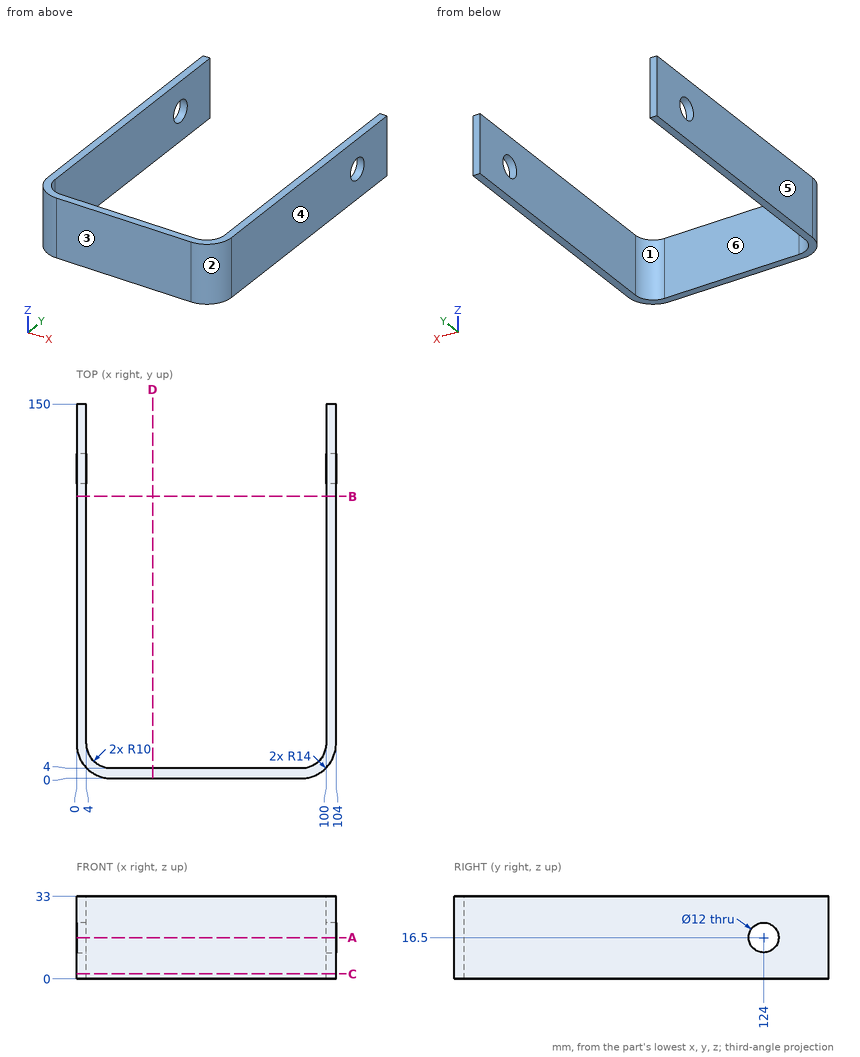
Here's the drawing with two shaded views (mm, measured from the low corner). I have some questions. A direction names the side the tool comes from. Give positions to 0.01 mm unless a question says otherwise; leave off trailing zeros. Order: outer loops, then holes, each group sorted by start corner. A loop starts at its lowest first (then second) coordinate and runs counter-clockwise, first axis right, second up. Notation, with made-up numbers: (60.25, 56) - (79.25, 56) arc R12 cw to (79.25, 75) - close; hole circle Ø8 at (20, 65). An arc over 180 degrees is marked (long way). Use a Markdown table: item, result. Add a question column.
Q1. If we mould it in two halves opening along X, with no side actions, what happens to the marked faces 3, 4, 5 and 6? For each: released by +X, released by -X, zero draft, split by the parting line, or undercut.
Q2. If we section it at A-A on z = 16.5: Write out the boundary of the cut face in (x, y), plus the area to 3 significant figures.
Q3. If we section it at B-B on y = 113: Write out the boundary of the cut face in (x, z), plus the area to 3 significant figures.
Q4. I'm going to push a flat-ended pin straight in: pin 1 (2 mm diameter, centred on x = 69, z = 13.5, fed in from +Y). Where does the tip first touch, or does it pass through?
Q5. If we section it at D-D on x = 30.5: Write out the boundary of the cut face in (y, z), plus the area to 3 significant figures.
Q6. On a 3-axis mill with a long thin cutter (end or side, diameter ignored), from which of +Z, -Z, +X, -X, +Y, -Y can I reach the whole of each face in a straight line? I mean the marked faces 1 and 2. Say none if no direction works.
Q7. If we section it at C-C on z = 2: Write out the boundary of the cut face in (x, y), plus the area to 3 significant figures.
Q8. Please list where these lines run through material, in increasing order: line 1 along X through (y, z) = (102.5, 31); line 2 along Z through (x, y) = (101.55, 124); line 3 along Y through (x, z) = (54, 16).
Answers follow:
| question | item | result |
|---|---|---|
| 1 | face 3 | zero draft |
| 1 | face 4 | released by +X |
| 1 | face 5 | released by -X |
| 1 | face 6 | undercut |
| 2 | outline | (0, 14) arc R14 ccw to (14, 0) - (90, 0) arc R14 ccw to (104, 14) - (104, 118) - (100, 118) - (100, 14) arc R10 cw to (90, 4) - (14, 4) arc R10 cw to (4, 14) - (4, 118) - (0, 118) - close; (0, 130) - (4, 130) - (4, 150) - (0, 150) - close; (100, 130) - (104, 130) - (104, 150) - (100, 150) - close |
| 2 | area | 1,450 mm^2 |
| 3 | outline | (0, 0) - (4, 0) - (4, 33) - (0, 33) - close; (100, 0) - (104, 0) - (104, 33) - (100, 33) - close |
| 3 | area | 264 mm^2 |
| 4 | pin 1 | stops at y = 4 |
| 5 | outline | (0, 0) - (4, 0) - (4, 33) - (0, 33) - close |
| 5 | area | 132 mm^2 |
| 6 | face 1 | +Z, -Z, +Y |
| 6 | face 2 | +Z, -Z, +X, -Y |
| 7 | outline | (0, 14) arc R14 ccw to (14, 0) - (90, 0) arc R14 ccw to (104, 14) - (104, 150) - (100, 150) - (100, 14) arc R10 cw to (90, 4) - (14, 4) arc R10 cw to (4, 14) - (4, 150) - (0, 150) - close |
| 7 | area | 1,540 mm^2 |
| 8 | line 1 | x = 0 to 4, 100 to 104 |
| 8 | line 2 | z = 0 to 10.5, 22.5 to 33 |
| 8 | line 3 | y = 0 to 4 |
